from build123d import *

# Parameters (mm, degrees)
PAD_DEPTH           = 10
SKETCH001_W         = 20
SKETCH001_H         = 2
POCKET_DEPTH        = 4
LINEARPATTERN_COUNT = 6
LINEARPATTERN_PITCH = 4
POCKET001_DEPTH     = 50
SKETCH003_R         = 1.75
POCKET002_DEPTH     = 10


with BuildPart() as part:
    # Sketch → Pad (new body, symmetric)
    with BuildSketch(Plane.XZ):
        with BuildLine():
            ThreePointArc((20, 0), (0, 20), (-20, 0))
            add(Edge.make_bspline(
                [(-20, 0), (-20, -20), (-15, -25), (-15, -40)],
                knots=[0, 0, 0, 0, 1, 1, 1, 1], degree=3))
            ThreePointArc((-15, -40), (0, -55), (15, -40))
            add(Edge.make_bspline(
                [(20, 0), (20, -20), (15, -25), (15, -40)],
                knots=[0, 0, 0, 0, 1, 1, 1, 1], degree=3))
        make_face()
    extrude(amount=PAD_DEPTH, both=True)

    # Sketch001 (on Face6 of Pad) → Pocket (cut)
    with BuildSketch(Plane.XZ.offset(10)):
        with Locations((0, 10)):
            Rectangle(SKETCH001_W, SKETCH001_H)
    pocket = extrude(amount=-POCKET_DEPTH, mode=Mode.SUBTRACT)

    # LinearPattern: Pocket ×6
    with Locations(*[(0, 0, -i * LINEARPATTERN_PITCH) for i in range(1, LINEARPATTERN_COUNT)]):
        add(pocket, mode=Mode.SUBTRACT)

    # Sketch002 → Pocket001 (cut, symmetric)
    with BuildSketch(Plane.YZ):
        with BuildLine():
            ThreePointArc((4, -5), (0, -1), (-4, -5))
            Line((-4, -5), (-4, -20))
            ThreePointArc((-4, -20), (0, -24), (4, -20))
            Line((4, -5), (4, -20))
        make_face()
    extrude(amount=POCKET001_DEPTH, both=True, mode=Mode.SUBTRACT)

    # Sketch003 → Pocket002 (cut)
    with BuildSketch(Plane.XY.offset(-55)):
        Circle(SKETCH003_R)
    extrude(amount=POCKET002_DEPTH, mode=Mode.SUBTRACT)


solid = part.part
CAD build for the part. Positions are in the model's coordinates, mm. A direction names the side the tool comes from. Coordinates: 2 decimals unless noted, no trailing zeros. Order: outer loops, then holes, each group sorted by start corner. A loop starts at its lowest first (then second) coordinate and runs counter-clockwise, first axis right, second up. Notation, with made-up numbers: (89.25, 32.5) -> (141.25, 32.5) arc R17 ccw to (141.25, 43.5) -> close; hole circle Ø11 at (57, 88). An arc over 180 degrees is marked (long way). Answer in a Markdown table with one row per item.
1) Mould opens along X. For faces 1 (the face through (0, -10, -17)), 2 (the face through (0, -8, -9)), 3 (the face through (0, -2, -55)) say: pulls with the +X half, pulls with the -X half, needs draft (parallel to the pull), parting line crosses it, or undercut.
Check values:
| item | result |
|---|---|
| face 1 | needs draft |
| face 2 | undercut |
| face 3 | parting line crosses it |
2) Flat gauge pins, fed straight in: P1, Ø5, axis at x = -11.5, y = -7.5, coming from the -Z side; P2, Ø1.5, axis at x = -14, y = -4, coming from the -Z side; P3, Ø1.5, axis at y = 0, z = -36, coming from the -X side. Where does each tip first touch, or does it go through?
Check values:
| item | result |
|---|---|
| P1 | z = -52 |
| P2 | z = -47.03 |
| P3 | x = -15.18 |
3) Which spindle directions (+Z, -Z, +X, -X, +Y, -Y) get a long thin tool onto all of the face, cutting with end or side? Do faces 4 (the face through (10, -8, 6)), 5 (the face through (0, 10, -17)), 6 (the face through (0, 0, -24)), 7 (the face through (0, 0, -45)). Say none if no direction does.
Check values:
| item | result |
|---|---|
| face 4 | -Y |
| face 5 | +Z, -Z, +X, -X, +Y |
| face 6 | +X, -X |
| face 7 | -Z |
4) Band-saw the part on B-B (x = 13.5). List the corners of the cut face in (y, z), and give its area (3 significant figures).
Check values:
| item | result |
|---|---|
| outline | (-10, -46.54) -> (10, -46.54) -> (10, 14.76) -> (-10, 14.76) -> close; hole (-4, -20) arc R4 ccw to (4, -20) -> (4, -5) arc R4 ccw to (-4, -5) -> close |
| area | 1,060 mm2 |
5) Drill centre lines: line 1 (Y direction, x = 0, z = -49.75); line 2 (Z direction, x = 10.5, y = 1); line 3 (X direction, y = 0, z = -48.75). Where is each one in solid material? Low to high.
Check values:
| item | result |
|---|---|
| line 1 | -10 to -1.75, 1.75 to 10 |
| line 2 | -50.71 to -23.87, -1.13 to 17.02 |
| line 3 | -12.18 to -1.75, 1.75 to 12.18 |
